Could you check a few things on this drawing? It's one solid part, dimensions in mm from its lowest x, y, z. Coordinates: 2 decimals unless noted, no trailing zeros. Loops run counter-clockwise (first coordinate to the right, second up) from the corner with the lowest first, then second, coordinate; pieces in that order, holes last. Notation, with made-up numbers: M 42.5,-21.75 L 52.5,-21.75 A30 cw 52.5,14.25 Z; hole C -10.75,-8.5 d11. An arc over 180 degrees is marked long. Answer as a JSON object with one key per item and string values. Group by question number.
Item 1: Suppose I cut it at A-A (y = 3). Write out the boundary of the cut face in (x, z).
Item 2: I'm going to push a flat-ended pin straight in: pin 1 Ø1.5 at (y, z) = (6, 5) entering from +X. Where does the tip first touch, or does it pass through?
Item 3: If I drill on line 1 (Y direction, x = 1.4, z = 0.55); line 2 (Y direction, x = 4.45, z = 4.65); line 3 (Z direction, x = 3.65, y = 6), over which ranges is the centre line in solid material (lowest first)?
Item 4: Suppose I cut it at B-B (y = 10). Write out the boundary of the cut face in (x, z).
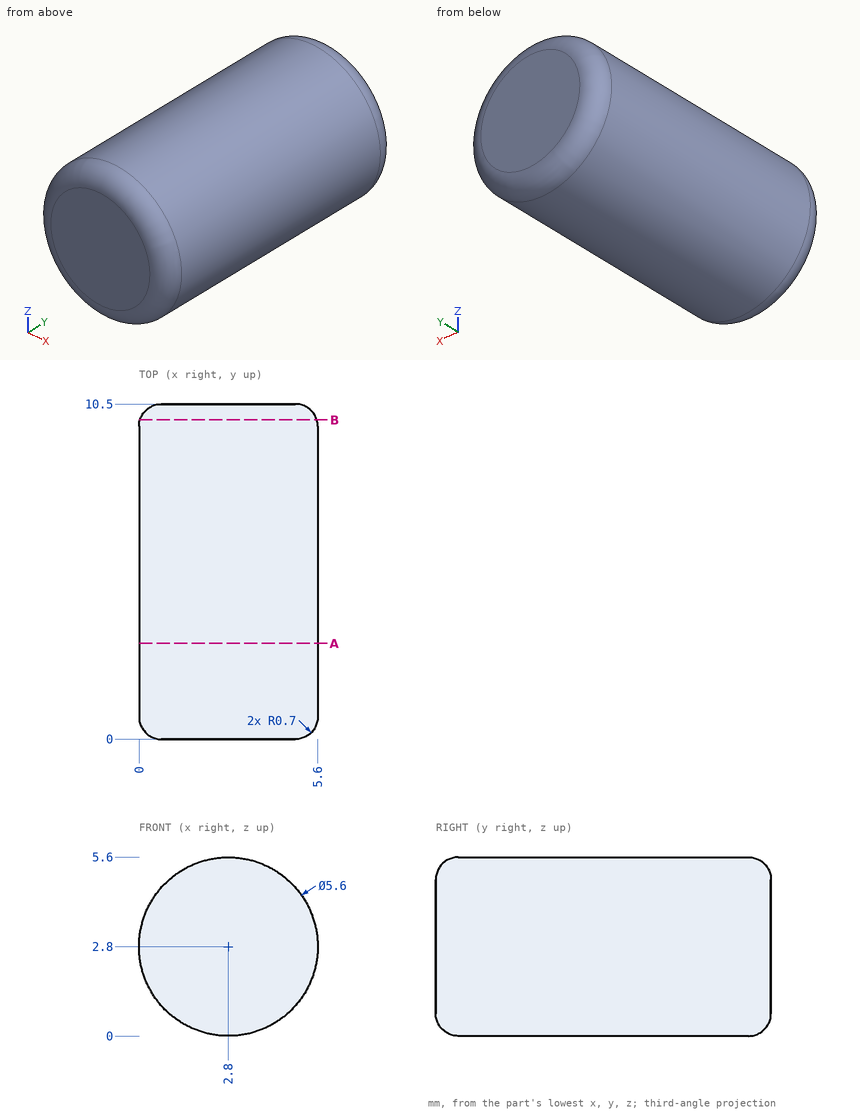
From the geometry:
{
 "1": {"outline": "C 2.8,2.8 d5.6"},
 "2": {"pin 1": "x = 5.2"},
 "3": {"line 1": "0.27 to 10.23", "line 2": "0.11 to 10.39", "line 3": "0.13 to 5.47"},
 "4": {"outline": "C 2.8,2.8 d5.54"}
}
